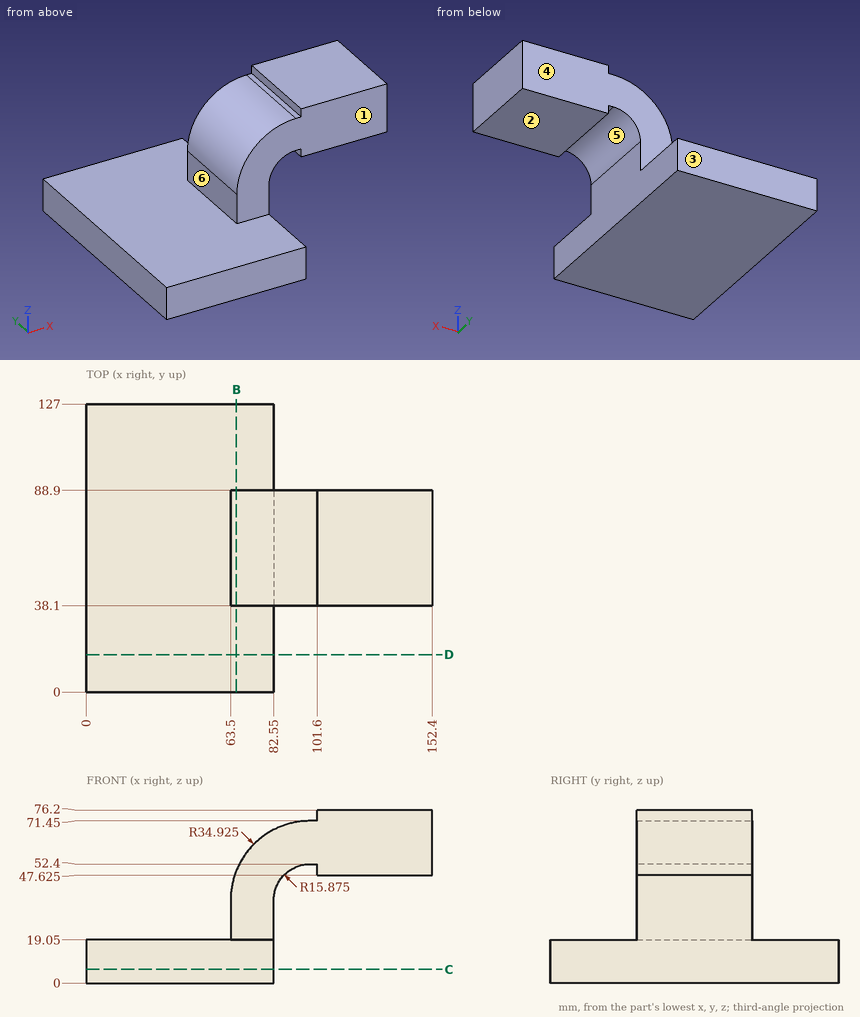
The drawing under review shows one solid part. Ordinate dimensions are in mm from its lowest x, y, z. A direction names the side the tool comes from. Round coordinates to 2 decimals unless told otherwise and drop trailing zeros. Write each loop counter-clockwise with the first axis right and the second up, starting at its lowest first coordinate (ties: lowest second). Pieces come first, ordered by that corner, then holes. Notation, with made-up numbers: (43, 62) - (83, 62) arc R20 ccw to (83, 70) - close; hole circle Ø5 at (2.5, 74). An arc over 180 degrees is marked (long way). Use a Markdown table: item, result. Add a question column.
1. We need section C-C (z = 6). State the section outline as (x, y) points.
2. We need section B-B (x = 66). State the section outline as (y, z) points.
3. For the marked faces 1, 2 and 3, list the 3-axis set-ups (+Z, -Z, +X, -X, +Y, -Y) from which the entire face can be reached by the end or side of a thin tool; tool diameter is ignored.
4. Mouldability with a two-part tool opening along X and no side actions: class the marked faces 4, 5 and 6 as +X half, -X half, draft (parallel to the pull), parting line (faces both ways), or undercut.
5. Clearance check with flat-ended pins moving along their axes: pin 1 (6 mm diameter, centred on x = 81, z = 32.5, fed in from +Y); pin 2 (1.5 mm diameter, centred on y = 74.5, z = 64.5, fed in from -X); pin 3 (2 mm diameter, centred on y = 72, z = 23, fed in from +X). State where each tip first meets the part, or that it passes through.
6. Wall thickness on probe 1 along Z at (x, y) = (73.5, 105); probe 2 along X at (y, z) = (53.5, 49.5); probe 3 along X at (y, z) = (41.5, 6): over which ranges is each line inside the solid? List them lowest first.
7. We need section D-D (y = 16.5). State the section outline as (x, z) points, then the cut area to 3 significant figures.
Output:
| question | item | result |
|---|---|---|
| 1 | outline | (0, 0) - (82.55, 0) - (82.55, 127) - (0, 127) - close |
| 2 | outline | (0, 0) - (127, 0) - (127, 19.05) - (88.9, 19.05) - (88.9, 49.5) - (38.1, 49.5) - (38.1, 19.05) - (0, 19.05) - close |
| 3 | face 1 | +Z, +X, -X, -Y |
| 3 | face 2 | -Z, +X, +Y, -Y |
| 3 | face 3 | +Z, -Z, +X, -X, +Y |
| 4 | face 4 | draft |
| 4 | face 5 | undercut |
| 4 | face 6 | -X half |
| 5 | pin 1 | stops at y = 88.9 |
| 5 | pin 2 | stops at x = 76.55 |
| 5 | pin 3 | stops at x = 82.55 |
| 6 | probe 1 | z = 0 to 19.05 |
| 6 | probe 2 | x = 66 to 89.28, 101.6 to 152.4 |
| 6 | probe 3 | x = 0 to 82.55 |
| 7 | outline | (0, 0) - (82.55, 0) - (82.55, 19.05) - (0, 19.05) - close |
| 7 | area | 1,570 mm2 |
